Input: part model. Units: mm. Frame: model coordinates. Round coordinates to 2 decimals unless told otherwise and drop trailing zeros. Loops run counter-clockwise (first coordinate to the right, second up) from the corner with the lowest first, then second, coordinate; pieces in that order, holes last. Notation, with made-up numbers: (-2, 16) - (50, 16) arc R16 cw to (50, 40) - close; hole circle Ø10 at (-36.75, 80). An arc over 180 degrees is marked (long way). One line per question, with ' | ' between items. Start each with the question number.
Item 1: First-contact query: pin 1 (1.5 mm diameter, centred on y = -10.5, z = 1.5, fed in from -X); pin 2 (1.5 mm diameter, centred on y = -39, z = 1, fed in from +X); pin 3 (1.5 mm diameter, centred on y = -40.5, z = 1.5, fed in from -X). Flat tips, straight axial feed; report the tip coordinate or a pass-through.
Item 2: Material intervals for line 1 along X through (y, z) = (5.5, 0.75); line 2 along X through (y, z) = (-15, 2.8); line 3 along Y through (x, z) = (-322.5, 2.3), sorted ascending.
Item 3: Section A-A, the plane x = 89.5. Return loops of the section in (y, z), plus the area to 4 significant figures.
Autodesk Inventor part; units mm, degrees
ref_plane "YZ Plane" through (0, 0, 0) normal (1, 0, 0) x (0, 1, 0)
ref_plane "XZ Plane" through (0, 0, 0) normal (0, 1, 0) x (-1, 0, 0)
ref_plane "XY Plane" through (0, 0, 0) normal (0, 0, 1) x (1, 0, 0)
sketch "Эскиз1" plane through (0, 0, 0) normal (0, 0, 1) x (1, 0, 0)
  line L0 (-367, -44.25) -> (367, -44.25)
  line L1 (367, -44.25) -> (367, 44.25)
  line L2 (367, 44.25) -> (-367, 44.25)
  line L3 (-367, 44.25) -> (-367, -44.25)
  line L4 (-367, -44.25) -> (367, 44.25) construction
  line L5 (367, -44.25) -> (-367, 44.25) construction
  point P0 (0, 0)
  dimension "d0" = 734
  dimension "d1" = 88.5
extrude "Выдавливание1" add sketch "Эскиз1" along normal blind 3
sketch "Эскиз2" plane through (0, 0, 3) normal (0, 0, 1) x (1, 0, 0)
  line L0 (-367, -44.25) -> (367, -44.25)
  line L1 (-367, -44.25) -> (-351, -44.25)
  line L2 (-351, -44.25) -> (-351, -36.25)
  line L3 (-351, -36.25) -> (-367, -36.25)
  line L4 (-367, -36.25) -> (-367, -44.25)
  line L5 (-335, -44.25) -> (-319, -44.25)
  line L6 (-319, -44.25) -> (-319, -36.25)
  line L7 (-319, -36.25) -> (-335, -36.25)
  line L8 (-335, -36.25) -> (-335, -44.25)
  line L9 (-303, -44.25) -> (-287, -44.25)
  line L10 (-287, -44.25) -> (-287, -36.25)
  line L11 (-287, -36.25) -> (-303, -36.25)
  line L12 (-303, -36.25) -> (-303, -44.25)
  line L13 (-271, -44.25) -> (-255, -44.25)
  line L14 (-255, -44.25) -> (-255, -36.25)
  line L15 (-255, -36.25) -> (-271, -36.25)
  line L16 (-271, -36.25) -> (-271, -44.25)
  line L17 (-239, -44.25) -> (-223, -44.25)
  line L18 (-223, -44.25) -> (-223, -36.25)
  line L19 (-223, -36.25) -> (-239, -36.25)
  line L20 (-239, -36.25) -> (-239, -44.25)
  line L21 (-207, -44.25) -> (-191, -44.25)
  line L22 (-191, -44.25) -> (-191, -36.25)
  line L23 (-191, -36.25) -> (-207, -36.25)
  line L24 (-207, -36.25) -> (-207, -44.25)
  line L25 (-175, -44.25) -> (-159, -44.25)
  line L26 (-159, -44.25) -> (-159, -36.25)
  line L27 (-159, -36.25) -> (-175, -36.25)
  line L28 (-175, -36.25) -> (-175, -44.25)
  line L29 (-143, -44.25) -> (-127, -44.25)
  line L30 (-127, -44.25) -> (-127, -36.25)
  line L31 (-127, -36.25) -> (-143, -36.25)
  line L32 (-143, -36.25) -> (-143, -44.25)
  line L33 (-111, -44.25) -> (-95, -44.25)
  line L34 (-95, -44.25) -> (-95, -36.25)
  line L35 (-95, -36.25) -> (-111, -36.25)
  line L36 (-111, -36.25) -> (-111, -44.25)
  line L37 (-79, -44.25) -> (-63, -44.25)
  line L38 (-63, -44.25) -> (-63, -36.25)
  line L39 (-63, -36.25) -> (-79, -36.25)
  line L40 (-79, -36.25) -> (-79, -44.25)
  line L41 (-47, -44.25) -> (-31, -44.25)
  line L42 (-31, -44.25) -> (-31, -36.25)
  line L43 (-31, -36.25) -> (-47, -36.25)
  line L44 (-47, -36.25) -> (-47, -44.25)
  line L45 (-15, -44.25) -> (1, -44.25)
  line L46 (1, -44.25) -> (1, -36.25)
  line L47 (1, -36.25) -> (-15, -36.25)
  line L48 (-15, -36.25) -> (-15, -44.25)
  line L49 (17, -44.25) -> (33, -44.25)
  line L50 (33, -44.25) -> (33, -36.25)
  line L51 (33, -36.25) -> (17, -36.25)
  line L52 (17, -36.25) -> (17, -44.25)
  line L53 (49, -44.25) -> (65, -44.25)
  line L54 (65, -44.25) -> (65, -36.25)
  line L55 (65, -36.25) -> (49, -36.25)
  line L56 (49, -36.25) -> (49, -44.25)
  line L57 (81, -44.25) -> (97, -44.25)
  line L58 (97, -44.25) -> (97, -36.25)
  line L59 (97, -36.25) -> (81, -36.25)
  line L60 (81, -36.25) -> (81, -44.25)
  line L61 (113, -44.25) -> (129, -44.25)
  line L62 (129, -44.25) -> (129, -36.25)
  line L63 (129, -36.25) -> (113, -36.25)
  line L64 (113, -36.25) -> (113, -44.25)
  line L65 (145, -44.25) -> (161, -44.25)
  line L66 (161, -44.25) -> (161, -36.25)
  line L67 (161, -36.25) -> (145, -36.25)
  line L68 (145, -36.25) -> (145, -44.25)
  line L69 (177, -44.25) -> (193, -44.25)
  line L70 (193, -44.25) -> (193, -36.25)
  line L71 (193, -36.25) -> (177, -36.25)
  line L72 (177, -36.25) -> (177, -44.25)
  line L73 (209, -44.25) -> (225, -44.25)
  line L74 (225, -44.25) -> (225, -36.25)
  line L75 (225, -36.25) -> (209, -36.25)
  line L76 (209, -36.25) -> (209, -44.25)
  line L77 (241, -44.25) -> (257, -44.25)
  line L78 (257, -44.25) -> (257, -36.25)
  line L79 (257, -36.25) -> (241, -36.25)
  line L80 (241, -36.25) -> (241, -44.25)
  line L81 (273, -44.25) -> (289, -44.25)
  line L82 (289, -44.25) -> (289, -36.25)
  line L83 (289, -36.25) -> (273, -36.25)
  line L84 (273, -36.25) -> (273, -44.25)
  line L85 (305, -44.25) -> (321, -44.25)
  line L86 (321, -44.25) -> (321, -36.25)
  line L87 (321, -36.25) -> (305, -36.25)
  line L88 (305, -36.25) -> (305, -44.25)
  line L89 (337, -44.25) -> (353, -44.25)
  line L90 (353, -44.25) -> (353, -36.25)
  line L91 (353, -36.25) -> (337, -36.25)
  line L92 (337, -36.25) -> (337, -44.25)
  point P0 (0, 0)
  dimension "d4" = 16
  dimension "d5" = 8
  dimension "d8" = 32
extrude "Выдавливание2" cut sketch "Эскиз2" against normal blind 3
sketch "Эскиз3" plane through (0, 0, 3) normal (0, 0, 1) x (1, 0, 0)
  line L0 (367, 44.25) -> (-367, 44.25)
  line L1 (-367, 44.25) -> (-370, 44.25)
  line L2 (-370, 44.25) -> (-370, 28.25)
  line L3 (-370, 28.25) -> (-367, 28.25)
  line L4 (-367, 28.25) -> (-367, 44.25)
  line L5 (-367, 12.25) -> (-370, 12.25)
  line L6 (-370, 12.25) -> (-370, -3.75)
  line L7 (-370, -3.75) -> (-367, -3.75)
  line L8 (-367, -3.75) -> (-367, 12.25)
  line L9 (-367, -19.75) -> (-370, -19.75)
  line L10 (-370, -19.75) -> (-370, -35.75)
  line L11 (-370, -35.75) -> (-367, -35.75)
  line L12 (-367, -35.75) -> (-367, -19.75)
  line L13 (367, -44.25) -> (367, 44.25)
  line L14 (367, 28.25) -> (367, 44.25)
  line L15 (367, 28.25) -> (370, 28.25)
  line L16 (370, 28.25) -> (370, 12.25)
  line L17 (370, 12.25) -> (367, 12.25)
  line L18 (367, 12.25) -> (367, 28.25)
  line L19 (370, -19.75) -> (367, -19.75)
  line L20 (370, -3.75) -> (370, -19.75)
  line L21 (367, -3.75) -> (370, -3.75)
  line L22 (367, -19.75) -> (367, -3.75)
  point P0 (0, 0)
  dimension "d15" = 3
  dimension "d16" = 16
  dimension "d19" = 32
  dimension "d24" = 3
  dimension "d25" = 16
  dimension "d28" = 32
extrude "Выдавливание3" add sketch "Эскиз3" against normal blind 3
properties part number "КВ33.044.004 - Стенка блока управления" material "Дерево (береза)"
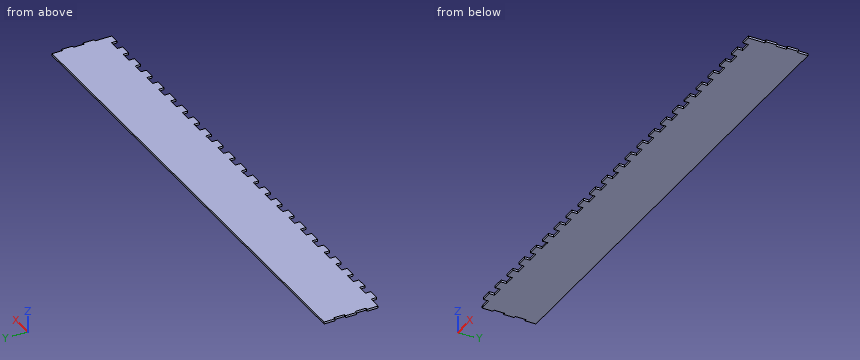
Return value:
1) pin 1: x = -367 | pin 2: x = 367 | pin 3: x = -351
2) line 1: -370 to 367 | line 2: -367 to 370 | line 3: -36.25 to 44.25
3) outline: (-36.25, 0) - (44.25, 0) - (44.25, 3) - (-36.25, 3) - close | area: 241.5 mm2
